The figure shows three views and two pictorial views of one solid part (mm, origin at its lowest corner). Answer the questions. Round coordinates to 2 decimals unless told otherwise and drop trailing zeros. Order: outer loops, then holes, each group sorted by start corner. A loop starts at its lowest first (then second) coordinate and runs counter-clockwise, first axis right, second up. Notation, with made-up numbers: (-37.75, 44) - (-31.75, 44) arc R9 cw to (-31.75, 50) - close; hole circle Ø10 at (64.5, 44). An arc over 180 degrees is marked (long way). Use CSV: the item, a comma, the result in double quotes.
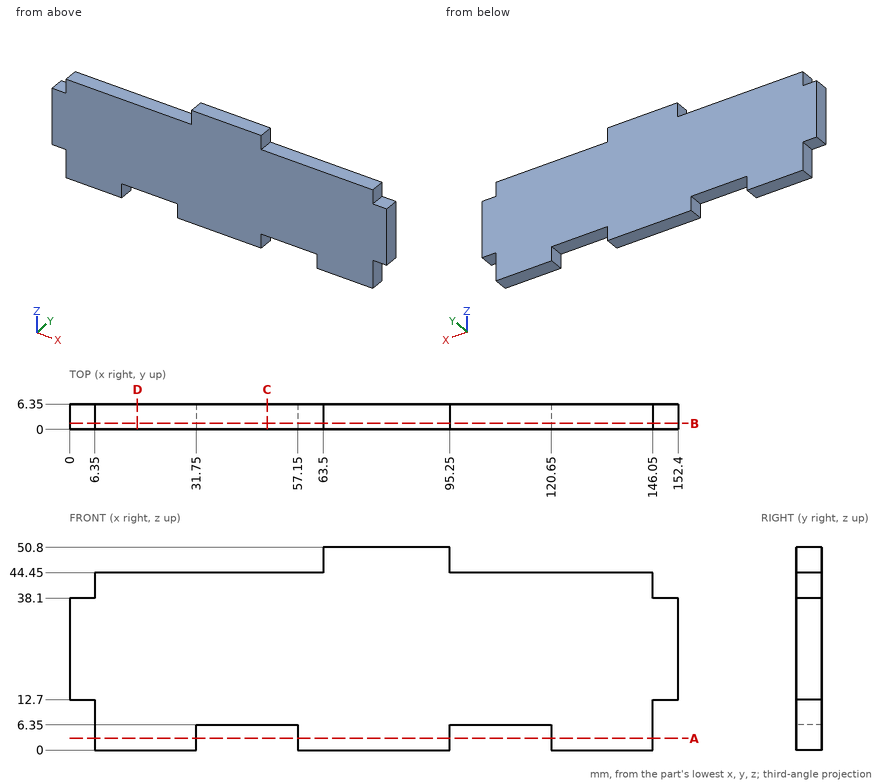
(1) Find the intervals of material crossed by L1, parallel to X at y = 3.75, z = 5; L2, parallel to X at y = 4, z = 38.5; L3, parallel to Z at x = 48.5, y = 5, in increasing order. Write a range as from..to.
Findings below:
L1,"x = 6.35..31.75, 57.15..95.25, 120.65..146.05"
L2,"x = 6.35..146.05"
L3,"z = 6.35..44.45"
(2) Find section C-C (x = 49.5). Determine the outline of the cut face in (y, z).
Findings below:
outline,"(0, 6.35) - (6.35, 6.35) - (6.35, 44.45) - (0, 44.45) - close"
(3) Find section D-D (x = 17). Determine the outline of the cut face in (y, z), and give its area (3 significant figures).
Findings below:
outline,"(0, 0) - (6.35, 0) - (6.35, 44.45) - (0, 44.45) - close"
area,"282 mm²"
(4) Each of these flat-tipped pins is pushed along its axis until it touches: pin 1 (3 mm diameter, centred on x = 118, y = 4.5, fed in from +Z); pin 2 (3 mm diameter, centred on x = 150, y = 4, fed in from -Z); pin 3 (1.9 mm diameter, centred on y = 4, z = 1.5, fed in from +X). Where does it stop, or does it pass through?
Findings below:
pin 1,"stops at z = 44.45"
pin 2,"stops at z = 12.7"
pin 3,"stops at x = 146.05"
(5) Find section B-B (y = 1.5). Determine the outline of the cut face in (x, z).
Findings below:
outline,"(0, 12.7) - (6.35, 12.7) - (6.35, 0) - (31.75, 0) - (31.75, 6.35) - (57.15, 6.35) - (57.15, 0) - (95.25, 0) - (95.25, 6.35) - (120.65, 6.35) - (120.65, 0) - (146.05, 0) - (146.05, 12.7) - (152.4, 12.7) - (152.4, 38.1) - (146.05, 38.1) - (146.05, 44.45) - (95.25, 44.45) - (95.25, 50.8) - (63.5, 50.8) - (63.5, 44.45) - (6.35, 44.45) - (6.35, 38.1) - (0, 38.1) - close"
(6) Find section A-A (z = 3). Determine the outline of the cut face in (x, y).
Findings below:
outline,"(6.35, 0) - (31.75, 0) - (31.75, 6.35) - (6.35, 6.35) - close; (57.15, 0) - (95.25, 0) - (95.25, 6.35) - (57.15, 6.35) - close; (120.65, 0) - (146.05, 0) - (146.05, 6.35) - (120.65, 6.35) - close"
